from build123d import *

# Parameters (mm, degrees)
SKETCH1_R          = 4.0005
SKETCH1_R_2        = 2.54
EXTRUDE1_DEPTH     = 0.762
SKETCH2_R          = 3.175
SKETCH2_R_2        = 2.54
EXTRUDE2_DEPTH     = 3.429
CUT_EXTRUDE1_DEPTH = 5.318


with BuildPart() as part:
    # Sketch1 → Extrude1 (new body)
    with BuildSketch(Plane(origin=(0, 0, 0), x_dir=(1, 0, 0), z_dir=(0, 1, 0))):
        Circle(SKETCH1_R)
        Circle(SKETCH1_R_2, mode=Mode.SUBTRACT)
    extrude(amount=-EXTRUDE1_DEPTH)

    # Sketch2 → Extrude2 (add)
    with BuildSketch(Plane.XZ.offset(0.762)):
        Circle(SKETCH2_R)
        Circle(SKETCH2_R_2, mode=Mode.SUBTRACT)
    extrude(amount=EXTRUDE2_DEPTH)

    # Sketch3 → Revolve1 (revolve)
    with BuildSketch(Plane(origin=(0, 0, 0), x_dir=(0, 0, -1), z_dir=(1, 0, 0))):
        Polygon((-3.175, -4.191), (-2.54, -4.191), (-2.921, -4.826), (-2.54, -6.858), (-3.175, -6.858), (-3.556, -4.826), align=None)
    revolve(axis=Axis((0, 1.21490396, 0), (0, -1, 0)))

    # Sketch5 → Cut-Extrude1 (cut, through all)
    with BuildSketch(Plane.XZ.offset(2.54)):
        Polygon((-0.254, 0.254), (-4.064, 0.254), (-4.064, -0.254), (-0.254, -0.254), (-0.254, -4.064), (0.254, -4.064), (0.254, -0.254), (4.064, -0.254), (4.064, 0.254), (0.254, 0.254), (0.254, 4.064), (-0.254, 4.064), align=None)
    extrude(amount=CUT_EXTRUDE1_DEPTH, mode=Mode.SUBTRACT)


solid = part.part
For this review, take the finished solid that the model builds, in its own axes (mm). A direction names the side the tool comes from. Give positions to 0.01 mm unless a question says otherwise; leave off trailing zeros. Order: outer loops, then holes, each group sorted by start corner. A loop starts at its lowest first (then second) coordinate and runs counter-clockwise, first axis right, second up. Notation, with made-up numbers: (88, 73) - (97, 73) arc R25 ccw to (97, 103) - close; hole circle Ø10 at (-15, 4.25). An arc over 180 degrees is marked (long way). Answer as a JSON object with one key per item and string values. Group by question number.
Item 1: Draft analysis for pull direction X (two halves, no side actions). For faces 1 (the cylindrical face through (-0.9, -0.4, 3.9)), 2 (the conical face through (1.92, -4.44, 1.88)), 3 (the conical face through (2.29, -4.36, -2.34)), state which applies: pulls with the +X half, pulls with the -X half, needs draft (parallel to the pull), parting line crosses it, or undercut.
Item 2: Take a section at A-A on y = -4. Give the boundary of the cut face in (x, z) (3 decimals), and give its area (3 significant figures).
Item 3: Machinability: for faces 4 (the flat face through (-0.254, -4.67, 3.04)), 5 (the conical face through (2.34, -4.36, 2.29)), 6 (the conical face through (-1.92, -4.44, -1.88)), 7 (the flat face through (-3.04, -4.67, -0.254)), which of the approach directions +Z, -Z, +X, -X, +Y, -Y give a long, thin tool a straight path to every point of the face, cutting with its end or side? Answer none if there is none.
Item 4: Take a section at B-B on z = 0. Give the boundary of the cut face in (x, y) (1 decimal).
Item 5: Clearance check with flat-ended pins moving along their axes: pin 1 Ø3 at (y, z) = (-3, 1) entering from +X; pin 2 Ø4 at (y, z) = (-1.5, -3) entering from -X; pin 3 Ø4 at (x, z) = (0, 0) entering from +Y; pin 4 Ø0.8 at (y, z) = (-4.5, 3) entering from -X. State where each tip first meets the part, or that it passes through.
Item 6: Wall thickness on line 1 along X through (y, z) = (-0.3, 0); line 2 along Z through (x, y) = (0, -1.65) (3 decimals): over which ranges is each line inside the solid? List them lowest first.
Item 7: Take a section at C-C on x = 0. Give the boundary of the cut face in (y, z) (1 decimal), and give its area (3 significant figures).
Reported:
{
 "1": {"face 1": "parting line crosses it", "face 2": "undercut", "face 3": "pulls with the +X half"},
 "2": {"outline": "(-3.165, -0.254) arc R3.175 ccw to (-0.254, -3.165) - (-0.254, -2.527) arc R2.54 cw to (-2.527, -0.254) - close; (-3.165, 0.254) - (-2.527, 0.254) arc R2.54 cw to (-0.254, 2.527) - (-0.254, 3.165) arc R3.175 ccw to start; (0.254, -3.165) arc R3.175 ccw to (3.165, -0.254) - (2.527, -0.254) arc R2.54 cw to (0.254, -2.527) - close; (0.254, 2.527) arc R2.54 cw to (2.527, 0.254) - (3.165, 0.254) arc R3.175 ccw to (0.254, 3.165) - close", "area": "10.1 mm^2"},
 "3": {"face 4": "+Z, -Z, -Y", "face 5": "+Z, +X", "face 6": "none", "face 7": "+X, -X, -Y"},
 "4": {"outline": "(-4, -0.8) - (-3.2, -0.8) - (-3.2, -2.5) - (-2.5, -2.5) - (-2.5, 0) - (-4, 0) - close; (2.5, -2.5) - (3.2, -2.5) - (3.2, -0.8) - (4, -0.8) - (4, 0) - (2.5, 0) - close"},
 "5": {"pin 1": "x = 3.27", "pin 2": "x = -3.83", "pin 3": "through", "pin 4": "x = -2.26"},
 "6": {"line 1": "-4 to -2.54, 2.54 to 4", "line 2": "-3.175 to -2.54, 2.54 to 3.175"},
 "7": {"outline": "(-2.5, -3.2) - (-0.8, -3.2) - (-0.8, -4) - (0, -4) - (0, -2.5) - (-2.5, -2.5) - close; (-2.5, 2.5) - (0, 2.5) - (0, 4) - (-0.8, 4) - (-0.8, 3.2) - (-2.5, 3.2) - close", "area": "4.48 mm^2"}
}
